Input: part model. Units: mm. Frame: model coordinates. Coordinates: 2 decimals unless noted, no trailing zeros. Write each loop counter-clockwise with the first axis right and the second up, starting at its lowest first coordinate (ties: lowest second). Pieces come first, ordered by that corner, then holes. Notation, with made-up numbers: (26.25, -26) - (74.25, -26) arc R20 ccw to (74.25, 3) - close; hole circle Ø7 at (50.5, -5.5). An arc over 180 degrees is marked (long way). Use a Markdown table: item, result. Add a question column.
Q1. Material intervals for probe 1 along X at (y, z) = (78, 1.75); probe 2 along X at (y, z) = (72.5, 6.25); probe 3 along Y at (x, z) = (-8, 4.5), sorted ascending. Write a range as from..to.
Q2. Section query B-B (x = 0). Return the cut outline in (y, z), then the cut area to 3 significant figures.
Q3. Section query D-D (y = 90.5). Return the cut outline in (x, z).
Q4. Section query A-A (y = 44). Return the cut outline in (x, z).
Q5. Pin query (flat end, axial travel): P1, Ø3, axis at y = 53, z = 3, coming from the +X side; P2, Ø3, axis at x = -78.5, z = 4.5, coming from the +Y side; P3, Ø3, axis at y = 106.5, z = 1, coming from the -X side. Return the tip coordinate at first contact, or that it passes through.
Q6. Section query C-C (x = 23). Return the cut outline in (y, z), then the cut area to 3 significant figures.
from build123d import *

# Parameters (mm, degrees)
F1_DEPTH = 6.35
F3_DEPTH = 25.4
F4_R     = 12.7
F5_R     = 12.7
F6_W     = 6.604
F6_H     = 6.604
F7_DEPTH = 25.4
F8_R     = 5.08


with BuildPart() as f1:
    # F0 (on Top) → F1 (new body)
    with BuildSketch(Plane.XY):
        Polygon((0, 0), (88.9, 0), (88.9, 51.132088), (25.4, 152.4), (0, 152.4), (-25.4, 152.4), (-88.9, 51.132088), (-88.9, 0), align=None)
    extrude(amount=F1_DEPTH)

    # F2 (on face) → F3 (cut)
    with BuildSketch(Plane.XY.offset(6.35)):
        Polygon((26.336802, 127), (0, 127), (-26.336802, 127), (-43.016926, 100.399034), (0, 73.42529), (43.016926, 100.399034), align=None)
        Polygon((-69.85, 57.606446), (-69.85, 22.130749), (-5.976504, 22.130749), (-5.976504, 62.182597), (-49.763763, 89.639379), align=None)
        Polygon((5.976504, 22.130749), (69.85, 22.130749), (69.85, 57.606446), (49.763763, 89.639379), (5.976504, 62.182597), align=None)
    extrude(amount=-F3_DEPTH, mode=Mode.SUBTRACT)

    # F4
    f4_edges = [f1.edges().sort_by_distance(p)[0] for p in [
        (-25.4, 152.4, 3.175),
        (25.4, 152.4, 3.175),
        (88.9, 51.132088, 3.175),
        (-88.9, 51.132088, 3.175),
    ]]
    fillet(f4_edges, radius=F4_R)

    # F5
    f5_edges = [f1.edges().sort_by_distance(p)[0] for p in [
        (-43.016926, 100.399034, 3.175),
        (0, 73.42529, 3.175),
        (-26.336802, 127, 3.175),
        (26.336802, 127, 3.175),
        (43.016926, 100.399034, 3.175),
        (-49.763763, 89.639379, 3.175),
        (-69.85, 57.606446, 3.175),
        (-69.85, 22.130749, 3.175),
        (-5.976504, 22.130749, 3.175),
        (-5.976504, 62.182597, 3.175),
        (49.763763, 89.639379, 3.175),
        (69.85, 57.606446, 3.175),
        (69.85, 22.130749, 3.175),
        (5.976504, 22.130749, 3.175),
        (5.976504, 62.182597, 3.175),
    ]]
    fillet(f5_edges, radius=F5_R)

    # F6 (on face) → F7 (cut)
    with BuildSketch(Plane.XY.offset(6.35)):
        with Locations((-79.375, 44.45)):
            Rectangle(F6_W, F6_H)
        with Locations((-79.375, 12.7)):
            Rectangle(F6_W, F6_H)
        with Locations((79.375, 12.7)):
            Rectangle(F6_W, F6_H)
        with Locations((79.375, 44.45)):
            Rectangle(F6_W, F6_H)
    extrude(amount=-F7_DEPTH, mode=Mode.SUBTRACT)

    # F8
    f8_edges = [f1.edges().sort_by_distance(p)[0] for p in [
        (-88.9, 0, 3.175),
        (88.9, 0, 3.175),
    ]]
    fillet(f8_edges, radius=F8_R)


solid = f1.part
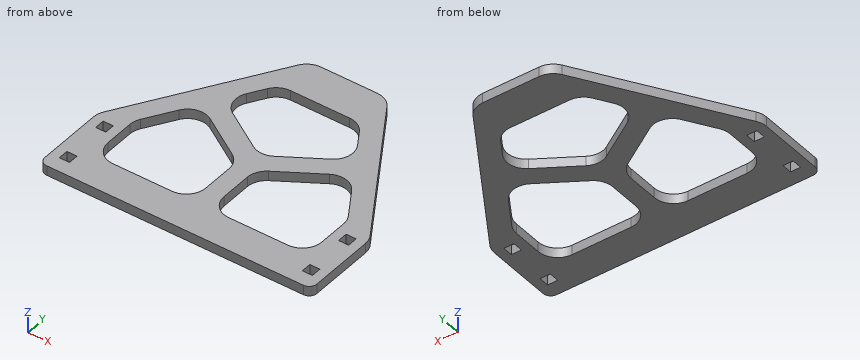
Values follow:
| question | item | result |
|---|---|---|
| 1 | probe 1 | -72.05..-57.06, -31.2..-7.3, 7.3..31.2, 57.06..72.05 |
| 1 | probe 2 | -75.5..-60.51, -22.43..22.43, 60.51..75.5 |
| 1 | probe 3 | 0..27.95, 62.03..78.44, 127..152.4 |
| 2 | outline | (0, 0) - (75.72, 0) - (75.72, 6.35) - (0, 6.35) - close; (127, 0) - (152.4, 0) - (152.4, 6.35) - (127, 6.35) - close |
| 2 | area | 642 mm2 |
| 3 | outline | (-64.21, 0) - (-27.23, 0) - (-27.23, 6.35) - (-64.21, 6.35) - close; (27.23, 0) - (64.21, 0) - (64.21, 6.35) - (27.23, 6.35) - close |
| 4 | outline | (-88.9, 0) - (-82.68, 0) - (-82.68, 6.35) - (-88.9, 6.35) - close; (-76.07, 0) - (-69.85, 0) - (-69.85, 6.35) - (-76.07, 6.35) - close; (-5.98, 0) - (5.98, 0) - (5.98, 6.35) - (-5.98, 6.35) - close; (69.85, 0) - (76.07, 0) - (76.07, 6.35) - (69.85, 6.35) - close; (82.68, 0) - (88.9, 0) - (88.9, 6.35) - (82.68, 6.35) - close |
| 5 | P1 | x = 88.25 |
| 5 | P2 | y = 70.11 |
| 5 | P3 | x = -55.12 |
| 6 | outline | (0, 0) - (22.13, 0) - (22.13, 6.35) - (0, 6.35) - close; (72.86, 0) - (87.85, 0) - (87.85, 6.35) - (72.86, 6.35) - close; (126.45, 0) - (151.53, 0) - (151.53, 6.35) - (126.45, 6.35) - close |
| 6 | area | 395 mm2 |
